The model under review builds one solid part; all positions refer to its coordinate system, in mm. Face numbers are marked on the shaded views. A direction names the side the tool comes from. Coordinates: 2 decimals unless noted, no trailing zeros. Loops run counter-clockwise (first coordinate to the right, second up) from the corner with the lowest first, then second, coordinate; pieces in that order, holes last. Notation, with made-up numbers: M -32,45 L 24,45 A29 cw 24,75 Z; hole C -17.5,38 d1. An arc over 180 degrees is marked long. Use one line per item in the form item = value.
```python
from build123d import *

# Parameters (mm, degrees)
F0_R            = 7.3279
F5_DEPTH        = 37.4904
F1_R            = 9.5377
F6_DEPTH        = 2.9972
F3_R            = 7.6073
F7_DEPTH        = 8.509
F4_R            = 5.9182
F8_DEPTH        = 17.5006
F9_SIZE         = 0.254
F11_D           = 9.525
F11_DEPTH       = 19.812
F11_TIP         = 2.8615986981
F13_D           = 4.2164
F17_D           = 3.5814
F17_DEPTH       = 6.35
F17_CSINK_D     = 5.08
F17_CSINK_ANGLE = 90
F17_TIP         = 1.0759611105


with BuildPart() as f5:
    # F0 (on Front) → F5 (new body)
    with BuildSketch(Plane.XZ):
        Circle(F0_R)
    extrude(amount=F5_DEPTH)

    # F1 (on Front) → F6 (join)
    with BuildSketch(Plane.XZ):
        Circle(F1_R)
    extrude(amount=-F6_DEPTH)

    # F3 (on Front) → F7 (join)
    with BuildSketch(Plane.XZ):
        Circle(F3_R)
    extrude(amount=-F7_DEPTH)

    # F4 (on Front) → F8 (join)
    with BuildSketch(Plane.XZ):
        Circle(F4_R)
    extrude(amount=-F8_DEPTH)

    # F9
    f9_edges = [f5.edges().sort_by_distance(p)[0] for p in [
        (-7.3279, -37.4904, 0),
        (-5.9182, 17.5006, 0),
    ]]
    chamfer(f9_edges, length=F9_SIZE)

    # F11
    with Locations(Plane.XZ.offset(37.4904)):
        with Locations((0, 0)):
            Hole(F11_D / 2, depth=F11_DEPTH)
            with Locations((0, 0, -(F11_DEPTH + F11_TIP / 2))):  # 118° drill point
                Cone(0, F11_D / 2, F11_TIP, mode=Mode.SUBTRACT)

    # F13 (through all)
    with Locations(Plane(origin=(0, 17.5006, 0), x_dir=(-1, 0, 0), z_dir=(0, 1, 0))):
        with Locations((0, 0)):
            Hole(F13_D / 2)

    # F17
    with Locations(Plane.YZ.offset(7.3279)):
        with Locations((-20.6248, 0)):
            CounterSinkHole(F17_D / 2, F17_CSINK_D / 2, depth=F17_DEPTH, counter_sink_angle=F17_CSINK_ANGLE)
            with Locations((0, 0, -(F17_DEPTH + F17_TIP / 2))):  # 118° drill point
                Cone(0, F17_D / 2, F17_TIP, mode=Mode.SUBTRACT)


solid = f5.part
```
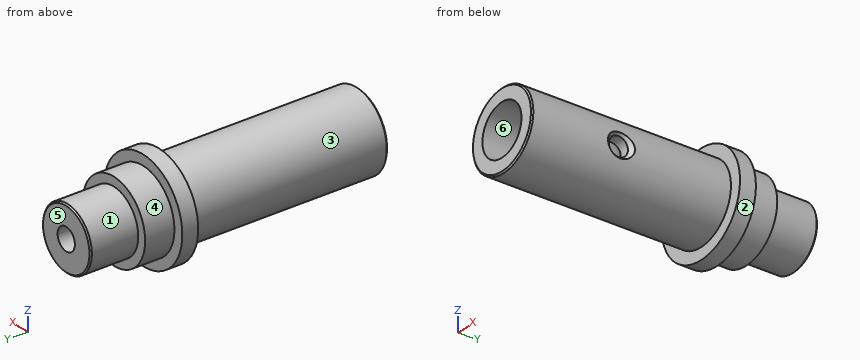
1. Add section A-A (x = 0). State the section outline as (y, z) points.
Response values:
outline = M -37.49,-7.07 L -37.24,-7.33 L 0,-7.33 L 0,-9.54 L 3,-9.54 L 3,-7.61 L 8.51,-7.61 L 8.51,-5.92 L 17.25,-5.92 L 17.5,-5.66 L 17.5,-2.11 L -16.08,-2.11 L -17.68,-4.76 L -37.49,-4.76 Z; M -37.49,4.76 L -17.68,4.76 L -16.08,2.11 L 17.5,2.11 L 17.5,5.66 L 17.25,5.92 L 8.51,5.92 L 8.51,7.61 L 3,7.61 L 3,9.54 L 0,9.54 L 0,7.33 L -37.24,7.33 L -37.49,7.07 Z
2. The part is to be moulded in two halves that separate along Z. For the marked faces 4, 5 and 6, say which applies: pulls with the +Z half, pulls with the -Z half, needs draft (parallel to the pull), parting line crosses it, or undercut.
Response values:
face_4 = parting line crosses it
face_5 = needs draft
face_6 = undercut
3. Machinability: for the marked faces 1, 2 and 3, which of the approach directions +Z, -Z, +X, -X, +Y, -Y give a long, thin tool a straight path to every point of the face, cutting with its end or side? Answer none if there is none.
Response values:
face_1 = +Y
face_2 = +Y, -Y
face_3 = -Y
4. Add section C-C (y = -4). State the section outline as (x, z) points.
Response values:
outline = C 0,0 d14.66; hole C 0,0 d4.22
5. Add section B-B (z = 0). Count the separate pieces of the cut face and the enclosed holes in it, then the cut area to 3 significant figures.
Response values:
separate_pieces = 3
enclosed_holes = 0
area = 446 mm^2
6. Wall thickness on line 1 along Z through (x, y) = (-0.25, -35); line 2 along Y through (x, z) = (5, 0); line 3 along Z through (x, y) = (0, -7.5): over which ranges is each line inside the solid? List them lowest first. Write a range as from..to.
Response values:
line_1 = -7.32..-4.76, 4.76..7.32
line_2 = -37.49..-22.42, -18.83..17.5
line_3 = -7.33..-2.11, 2.11..7.33
7. Insertion check: P1, Ø6, axis at y = 9.5, z = -3, coming from the -X side; P2, Ø3, axis at y = -20.62, z = 0, coming from the -X side; P3, Ø3, axis at y = -5, z = 6.5, coming from the -X side. Each pin has a flat end and moves straight along its axis. Give the tip position at first contact, or say it passes through.
Response values:
P1 = -7.61
P2 = -7.33
P3 = -5.36
8. Add section D-D (y = -28.5). State the section outline as (x, z) points (1 decimal).
Response values:
outline = C 0,0 d14.7; hole C 0,0 d9.5
